```python
from build123d import *

# Parameters (mm, degrees)
F0_R     = 14.2875
F1_DEPTH = 101.6
F2_R     = 15.875
F3_DEPTH = 12.7
F4_R     = 15.875
F5_DEPTH = 10.16
F7_DEPTH = 101.6


with BuildPart() as f1:
    # F0 (on Front) → F1 (new body)
    with BuildSketch(Plane.XZ):
        Circle(F0_R)
    extrude(amount=F1_DEPTH)

    # F2 (on face) → F3 (join)
    with BuildSketch(Plane.XZ.offset(101.6)):
        Circle(F2_R)
    extrude(amount=F3_DEPTH)

    # F4 (on face) → F5 (join)
    with BuildSketch(Plane(origin=(0, 0, 0), x_dir=(-1, 0, 0), z_dir=(0, 1, 0))):
        Circle(F4_R)
    extrude(amount=F5_DEPTH)

    # F6 (on Front) → F7 (cut)
    with BuildSketch(Plane.XZ):
        with BuildLine():
            Line((-14.2875, 0), (0, 0))
            Line((0, 0), (14.2875, 0))
            ThreePointArc((14.2875, 0), (0, 14.2875), (-14.2875, 0))
        make_face()
    extrude(amount=F7_DEPTH, mode=Mode.SUBTRACT)


solid = f1.part
```
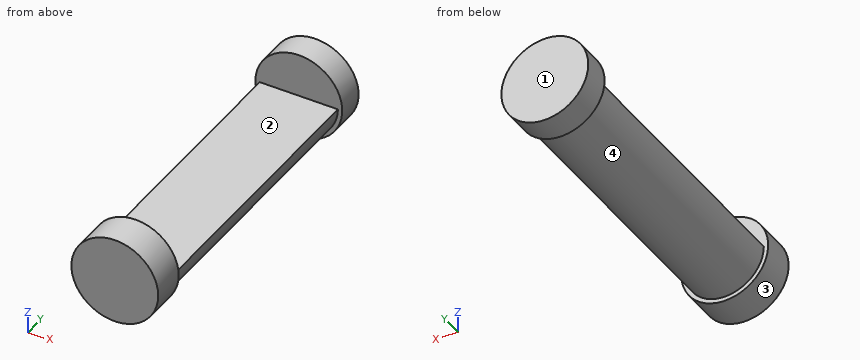
Geometry check sheet. Reference: the model listing, model coordinates, mm. Face numbers are marked on the shaded views. Give positions to 0.01 mm unless a question says otherwise; leave off trailing zeros. Order: outer loops, then holes, each group sorted by start corner. A loop starts at its lowest first (then second) coordinate and runs counter-clockwise, first axis right, second up.
1. Thickness scan on L1, parallel to Y at x = 3.5, z = 9; L2, parallel to Z at x = 0, y = -37; L3, parallel to Z at x = 3, y = 5. Record the ranges inside material, lowest first.
2. Release check for a two-part mould opening along Y. For the marked faces 1, 2, 3 and 4 record: pulls with the +Y half, pulls with the -Y half, needs draft (parallel to the pull), parting line crosses it, or undercut.
3. Section check A-A, the plane z = 2. Enter the section's corners in (x, y), and give its area (3 significant figures).
4. Section check C-C, the plane z = -8. Enter the section's corners in (x, y).
5. Section check D-D, the plane y = -22. Enter the section's corners in (x, z) (1 decimal).
6. Section check B-B, the plane x = 12. Enter the section's corners in (y, z).
7. Gauge pin test, flat ends, axial feed: pin 1 Ø5 at (y, z) = (-5, -8) entering from -X; pin 2 Ø8 at (x, y) = (7, -68.5) entering from +Z; pin 3 Ø6 at (x, y) = (11.5, -83) entering from -Z. Record the tip position at first contact, or that the pin passes through.
Values follow:
1. L1: y = -114.3 to -101.6, 0 to 10.16
1. L2: z = -14.29 to 0
1. L3: z = -15.59 to 15.59
2. face 1: pulls with the +Y half
2. face 2: undercut
2. face 3: needs draft
2. face 4: undercut
3. outline: (-15.75, -114.3) - (15.75, -114.3) - (15.75, -101.6) - (-15.75, -101.6) - close; (-15.75, 0) - (15.75, 0) - (15.75, 10.16) - (-15.75, 10.16) - close
3. area: 720 mm2
4. outline: (-13.71, -114.3) - (13.71, -114.3) - (13.71, -101.6) - (11.84, -101.6) - (11.84, 0) - (13.71, 0) - (13.71, 10.16) - (-13.71, 10.16) - (-13.71, 0) - (-11.84, 0) - (-11.84, -101.6) - (-13.71, -101.6) - close
5. outline: (-14.3, 0) arc R14.3 ccw to (14.3, 0) - close
6. outline: (-114.3, -10.39) - (-101.6, -10.39) - (-101.6, -7.75) - (0, -7.75) - (0, -10.39) - (10.16, -10.39) - (10.16, 10.39) - (0, 10.39) - (0, 0) - (-101.6, 0) - (-101.6, 10.39) - (-114.3, 10.39) - close
7. pin 1: stops at x = -13.19
7. pin 2: stops at z = 0
7. pin 3: stops at z = -11.48
